Build history of the part. All positions in model axes, mm. Round coordinates to 2 decimals unless told otherwise and drop trailing zeros. Order: outer loops, then holes, each group sorted by start corner. A loop starts at its lowest first (then second) coordinate and runs counter-clockwise, first axis right, second up. Notation, with made-up numbers: M 38.25,68 L 60.25,68 A32 cw 60.25,94 Z; hole C 80,-19 d8. An arc over 180 degrees is marked long. One line per item, written item: value. Start each with the question number.
Item 1: Band-saw the part on A-A, the plane z = -35.5. Write the cut outline in (x, y).
Item 2: Band-saw the part on C-C, the plane x = 16.25. Write the cut outline in (y, z), then the cut area to 3 significant figures.
Item 3: Probe L1, parallel to Z at x = 15, y = 1.25; L2, parallel to Z at x = 2.5, y = 4.5; L3, parallel to Y at x = 14.25, z = -36.25. List the from-to ranges inside material, lowest first.
Item 4: Band-saw the part on D-D, the plane y = 2. Write the cut outline in (x, z), then the cut area to 3 significant figures.
Item 5: Two-plate mould, pull along Z, no slides. Class faces 1 (the cylindrical face through (17.448, 1.232, -32.914)), 2 (the cylindrical face through (19.96, 1.23, -31.99)), 3 (the flat face through (13, 2.5, -35)): +Z half, -Z half, draft (parallel to the pull), parting line (faces both ways), or undercut.
Item 6: Pin check, flat tips, straight feed: pin 1 (6 mm diameter, centred on x = 15.5, z = -36, fed in from +Y); pin 2 (2.5 mm diameter, centred on x = 15.55, z = -34.12, fed in from +Y); pin 3 (1.5 mm diameter, centred on x = 2, y = 5.5, fed in from -Z). Stop position of each tip, or through.
```python
from build123d import *

# Parameters (mm, degrees)
SKETCH_1_R          = 4.9
SKETCH_1_R_2        = 2.25
EXTRUDE_1_DEPTH     = 10
CUT_EXTRUDE_START   = -7.5
SKETCH_2_R          = 2.25
CUT_EXTRUDE_1_DEPTH = 7.5


with BuildPart() as part:
    # ｽｹｯﾁ1 → ﾎﾞｽ - 押し出し1 (new body)
    # profile 1 of 3: a face of its own
    with BuildSketch(Plane(origin=(0, 0, 0), x_dir=(1, 0, 0), z_dir=(0, 1, 0))):
        with BuildLine():
            Line((8.453200419, 41.548807476), (6.499394662, 31.945545371))
            ThreePointArc((6.499394662, 31.945545371), (10.073954086, 31.004442409), (13.518999843, 29.66473737))
            ThreePointArc((13.518999843, 29.66473737), (11.092186389, 36.155544584), (17.582993695, 38.582357791))
            ThreePointArc((17.582993695, 38.582357791), (13.102320669, 40.324796256), (8.453200419, 41.548807476))
        make_face()
    # profile 2 of 3: a face of its own
    with BuildSketch(Plane(origin=(0, 0, 0), x_dir=(1, 0, 0), z_dir=(0, 1, 0))):
        with Locations((15.5509966, 34.123547658)):
            Circle(SKETCH_1_R)
        with Locations(Location((15.5509966, 34.123547658, 0), (0, 0, 270))):
            Circle(SKETCH_1_R_2, mode=Mode.SUBTRACT)
    # profile 3 of 3: a face of its own
    with BuildSketch(Plane(origin=(0, 0, 0), x_dir=(1, 0, 0), z_dir=(0, 1, 0))):
        with BuildLine():
            Line((0, 33.25), (0, 32.6))
            ThreePointArc((0, 32.6), (3.266130809, 32.435973695), (6.499394662, 31.945545371))
            Line((6.499394662, 31.945545371), (8.453200419, 41.548807476))
            ThreePointArc((8.453200419, 41.548807476), (4.247973812, 42.186665174), (0, 42.4))
            Line((0, 42.4), (0, 41.75))
            ThreePointArc((0, 41.75), (3.00520382, 40.50520382), (4.25, 37.5))
            ThreePointArc((4.25, 37.5), (3.00520382, 34.49479618), (0, 33.25))
        make_face()
    extrude(amount=EXTRUDE_1_DEPTH)

    # ｽｹｯﾁ2 → ｶｯﾄ - 押し出し1 (cut)
    with BuildSketch(Plane(origin=(0, 10, 0), x_dir=(1, 0, 0), z_dir=(0, 1, 0)).offset(CUT_EXTRUDE_START)):
        with BuildLine():
            ThreePointArc((13.518999843, 29.66473737), (20.00980681, 32.091550732), (17.582993695, 38.582357791))
            ThreePointArc((17.582993695, 38.582357791), (13.102320689, 40.32479625), (8.453200459, 41.548807468))
            ThreePointArc((8.453200459, 41.548807468), (12.277928583, 35.770273495), (6.499394603, 31.945545383))
            ThreePointArc((6.499394603, 31.945545383), (10.073954057, 31.004442418), (13.518999843, 29.66473737))
        make_face()
        with Locations(Location((15.5509966, 34.123547658, 0), (0, 0, 270))):
            Circle(SKETCH_2_R, mode=Mode.SUBTRACT)
    extrude(amount=CUT_EXTRUDE_1_DEPTH, mode=Mode.SUBTRACT)


solid = part.part
```
Output:
1. outline: M 3.75,0 L 13.77,0 L 13.77,2.5 L 12.21,2.5 L 12.21,10 L 3.75,10 Z; M 17.33,0 L 20.25,0 L 20.25,2.5 L 17.33,2.5 Z
2. outline: M 0,-39.16 L 2.5,-39.16 L 2.5,-36.26 L 0,-36.26 Z; M 0,-31.98 L 2.5,-31.98 L 2.5,-29.27 L 0,-29.27 Z
2. area: 14.0 mm²
3. L1: z = -39.66 to -36.31, -31.94 to -29.25
3. L2: z = -42.33 to -40.94, -34.06 to -32.5
3. L3: y = 0 to 2.5
4. outline: M 0,-42.4 A42.4 ccw 17.58,-38.58 A4.9 ccw 13.52,-29.66 A32.6 cw 0,-32.6 L 0,-33.25 A4.25 cw 0,-41.75 Z; hole C 15.55,-34.12 d4.5
4. area: 151 mm²
5. face 1: undercut
5. face 2: parting line
5. face 3: draft
6. pin 1: stops at y = 2.5
6. pin 2: passes through
6. pin 3: stops at z = -42.38
